Geometry: final body of the model. Coordinates: model frame, mm. Face numbers are marked on the shaded views. A direction names the side the tool comes from. Coordinates: 2 decimals unless noted, no trailing zeros. Order: outer loops, then holes, each group sorted by start corner. A loop starts at its lowest first (then second) coordinate and runs counter-clockwise, first axis right, second up. Notation, with made-up numbers: M -38,-19 L -3,-19 A21 ccw -3,-2 Z; hole C 27.5,86.5 d9. An arc over 180 degrees is marked long. One line per question, with ' | ' between items.
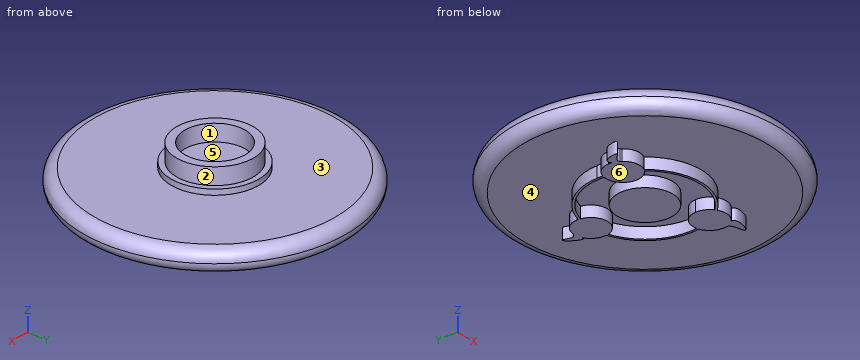
from build123d import *

# Parameters (mm, degrees)
SKETCH1_R           = 12
BOSS_EXTRUDE1_DEPTH = 2
SKETCH2_R           = 3.5
SKETCH2_R_2         = 2.75
BOSS_EXTRUDE2_DEPTH = 2
FILLET1_R           = 1
SKETCH3_R           = 2.5
BOSS_EXTRUDE3_DEPTH = 1
SKETCH4_R           = 3.992210858
BOSS_EXTRUDE4_DEPTH = 0.5


with BuildPart() as part:
    # Sketch1 → Boss-Extrude1 (new body)
    with BuildSketch(Plane.XY):
        Circle(SKETCH1_R)
    extrude(amount=BOSS_EXTRUDE1_DEPTH)

    # Sketch2 → Boss-Extrude2 (add)
    with BuildSketch(Plane.XY.offset(2)):
        Circle(SKETCH2_R)
        Circle(SKETCH2_R_2, mode=Mode.SUBTRACT)
    extrude(amount=BOSS_EXTRUDE2_DEPTH)

    # Fillet1
    fillet1_edges = [part.edges().sort_by_distance(p)[0] for p in [
        (-12, 0, 0),
        (-12, 0, 2),
    ]]
    fillet(fillet1_edges, radius=FILLET1_R - 0.0001)  # a hair under: the kernel refuses the full size

    # Sketch3 → Boss-Extrude3 (add)
    with BuildSketch(Plane(origin=(0, 0, 0), x_dir=(-1, 0, 0), z_dir=(0, 0, -1))):
        with Locations(Location((0, 0, 0), (0, 0, 180))):
            Circle(SKETCH3_R)
        with BuildLine():
            ThreePointArc((-5.067307925, -0.57653308), (-5.873937117, -1.230891086), (-6.062099925, -2.252375207))
            ThreePointArc((-6.062099925, -2.252375207), (-5.915680958, -2.687087026), (-5.644734338, -3.057223228))
            ThreePointArc((-5.644734338, -3.057223228), (-4.802200561, -3.480618607), (-3.873470329, -3.317563506))
            ThreePointArc((-3.873470329, -3.317563506), (-4.675755649, -2.036494318), (-5.067307925, -0.57653308))
        make_face()
        with BuildLine():
            ThreePointArc((-5.644734338, -3.057223228), (-5.915680958, -2.687087026), (-6.062099925, -2.252375207))
            add(Edge.make_bspline(
                [(-6.062099925, -2.252375207), (-6.026517589, -2.751047072), (-8.759907871, -2.687863498), (-5.681591245, -3.687002551), (-5.644734338, -3.057223228)],
                knots=[0, 0, 0, 0, 0.44427951, 1, 1, 1, 1], degree=3))
        make_face()
        with BuildLine():
            ThreePointArc((-1.49486588, 4.876), (-4.265918484, 2.794984703), (-5.067307925, -0.57653308))
            ThreePointArc((-5.067307925, -0.57653308), (-4.970460995, -0.547182079), (-4.871855436, -0.524427893))
            ThreePointArc((-4.871855436, -0.524427893), (-4.098627563, 2.68537746), (-1.464590045, 4.676))
            ThreePointArc((-1.464590045, 4.676), (-1.483103113, 4.775489073), (-1.49486588, 4.876))
        make_face()
        with BuildLine():
            ThreePointArc((-4.871855436, -0.524427893), (-4.970460995, -0.547182079), (-5.067307925, -0.57653308))
            ThreePointArc((-5.067307925, -0.57653308), (-4.675755649, -2.036494318), (-3.873470329, -3.317563506))
            ThreePointArc((-3.873470329, -3.317563506), (-3.786017441, -3.266643945), (-3.702196885, -3.209943649))
            ThreePointArc((-3.702196885, -3.209943649), (-4.492392683, -1.956631796), (-4.871855436, -0.524427893))
        make_face()
        with BuildLine():
            ThreePointArc((-3.702196885, -3.209943649), (-3.786017441, -3.266643945), (-3.873470329, -3.317563506))
            ThreePointArc((-3.873470329, -3.317563506), (0.01581793, -5.09997547), (3.893974917, -3.293472232))
            ThreePointArc((3.893974917, -3.293472232), (3.806118362, -3.243200717), (3.721809355, -3.187182945))
            ThreePointArc((3.721809355, -3.187182945), (0.015022472, -4.899976972), (-3.702196885, -3.209943649))
        make_face()
        with BuildLine():
            ThreePointArc((-3.084074166, -1.996563057), (-3.630573223, -0.838618346), (-4.871855436, -0.524427893))
            ThreePointArc((-4.871855436, -0.524427893), (-4.492392683, -1.956631796), (-3.702196885, -3.209943649))
            ThreePointArc((-3.702196885, -3.209943649), (-3.247508432, -2.677438992), (-3.084074166, -1.996563057))
        make_face()
        with BuildLine():
            ThreePointArc((1.49486588, 4.876), (0, 5.1), (-1.49486588, 4.876))
            ThreePointArc((-1.49486588, 4.876), (-1.483103113, 4.775489073), (-1.464590045, 4.676))
            ThreePointArc((-1.464590045, 4.676), (0, 4.9), (1.464590045, 4.676))
            ThreePointArc((1.464590045, 4.676), (1.483103113, 4.775489073), (1.49486588, 4.876))
        make_face()
        with BuildLine():
            ThreePointArc((-0.554469126, 6.393758942), (-1.275084916, 5.790036997), (-1.49486588, 4.876))
            ThreePointArc((-1.49486588, 4.876), (0, 5.1), (1.49486588, 4.876))
            ThreePointArc((1.49486588, 4.876), (1.49871592, 4.937946879), (1.5, 5))
            ThreePointArc((1.5, 5), (1.10747264, 6.011683919), (0.135327531, 6.493883014))
            ThreePointArc((0.135327531, 6.493883014), (-0.215467229, 6.484443961), (-0.554469126, 6.393758942))
        make_face()
        with BuildLine():
            ThreePointArc((5.074434577, -0.510013455), (4.695210635, -1.991230046), (3.893974917, -3.293472232))
            ThreePointArc((3.893974917, -3.293472232), (4.908886749, -3.438287773), (5.784206585, -2.904590527))
            add(Edge.make_bspline(
                [(5.865406446, -2.794015708), (5.836751545, -2.820305024), (5.809552866, -2.856598637), (5.784206585, -2.904590527)],
                knots=[0.961955758, 0.961955758, 0.961955758, 0.961955758, 1, 1, 1, 1], degree=3))
            ThreePointArc((5.865406446, -2.794015708), (6.004314758, -2.534169766), (6.090380192, -2.252375207))
            ThreePointArc((6.090380192, -2.252375207), (6.112856484, -2.103028092), (6.120373409, -1.952186319))
            ThreePointArc((6.120373409, -1.952186319), (5.831362343, -1.061421113), (5.074434577, -0.510013455))
        make_face()
        with BuildLine():
            ThreePointArc((3.721809355, -3.187182945), (3.806118362, -3.243200717), (3.893974917, -3.293472232))
            ThreePointArc((3.893974917, -3.293472232), (4.695210635, -1.991230046), (5.074434577, -0.510013455))
            ThreePointArc((5.074434577, -0.510013455), (4.97722395, -0.481798325), (4.878348324, -0.460127837))
            ThreePointArc((4.878348324, -0.460127837), (4.511084728, -1.913142593), (3.721809355, -3.187182945))
        make_face()
        with BuildLine():
            ThreePointArc((1.464590045, 4.676), (0, 4.9), (-1.464590045, 4.676))
            ThreePointArc((-1.464590045, 4.676), (0, 3.5), (1.464590045, 4.676))
        make_face()
        with BuildLine():
            add(Edge.make_bspline(
                [(-0.554469126, 6.393758942), (-1.437590662, 6.09502869), (0.002600213, 8.079848895), (-0.001852582, 7.193488902), (-0.442267062, 6.868197163), (0.135327531, 6.493883014)],
                knots=[0, 0, 0, 0, 0.556265111, 0.561970103, 1, 1, 1, 1], degree=3))
            ThreePointArc((-0.554469126, 6.393758942), (-0.215467229, 6.484443961), (0.135327531, 6.493883014))
        make_face()
        with BuildLine():
            ThreePointArc((5.1, 0), (4.100842352, 3.032011215), (1.49486588, 4.876))
            ThreePointArc((1.49486588, 4.876), (1.483103113, 4.775489073), (1.464590045, 4.676))
            ThreePointArc((1.464590045, 4.676), (3.948828385, 2.901164316), (4.9, 0))
            ThreePointArc((4.9, 0), (4.894584088, -0.230318487), (4.878348324, -0.460127837))
            ThreePointArc((4.878348324, -0.460127837), (4.97722395, -0.481798325), (5.074434577, -0.510013455))
            ThreePointArc((5.074434577, -0.510013455), (5.093604634, -0.255326906), (5.1, 0))
        make_face()
        with BuildLine():
            ThreePointArc((4.878348324, -0.460127837), (3.206344863, -1.359804857), (3.721809355, -3.187182945))
            ThreePointArc((3.721809355, -3.187182945), (4.511084728, -1.913142593), (4.878348324, -0.460127837))
        make_face()
        with BuildLine():
            ThreePointArc((6.090380192, -2.252375207), (6.004314758, -2.534169766), (5.865406446, -2.794015708))
            add(Edge.make_bspline(
                [(6.090380192, -2.252375207), (6.684980611, -1.62456302), (7.266645295, -4.471941038), (6.161555953, -2.52231461), (5.865406446, -2.794015708)],
                knots=[0, 0, 0, 0, 0.568767056, 0.961955758, 0.961955758, 0.961955758, 0.961955758], degree=3))
        make_face()
    extrude(amount=BOSS_EXTRUDE3_DEPTH)

    # Sketch4 → Boss-Extrude4 (add)
    with BuildSketch(Plane.XY.offset(2)):
        Circle(SKETCH4_R)
    extrude(amount=BOSS_EXTRUDE4_DEPTH)


solid = part.part
1. Pin query (flat end, axial travel): P1, Ø4, axis at x = -8, y = -6, coming from the -Z side; P2, Ø1.5, axis at x = -0.5, z = -0.5, coming from the -Y side; P3, Ø3, axis at x = 0.5, z = 3, coming from the +Y side. Return the tip coordinate at first contact, or that it passes through.
Response values:
P1: stops at z = 0 | P2: stops at y = -11.65 | P3: stops at y = 11.86
2. Section A-A, the plane z = 3.6. Output: boundary loops of the cut face in (x, y), and give its area (3 significant figures).
Response values:
outline: C 0,0 d7; hole C 0,0 d5.5 | area: 14.7 mm^2
3. Draft query along X for the marked faces 1, 2 and 3. Return one class per face: pulls with the +X half, pulls with the -X half, needs draft (parallel to the pull), parting line crosses it, or undercut.
Response values:
face 1: undercut | face 2: parting line crosses it | face 3: needs draft
4. Section B-B, the plane z = 1.5. Output: boundary loops of the cut face in (x, y), and give its area (3 significant figures).
Response values:
outline: C 0,0 d23.73 | area: 442 mm^2
5. Material intervals for line 1 (X direction, y = 0, z = 2.9); line 2 (X direction, y = 2, z = -0.3), sorted ascending. Write a range as [from, to].
Response values:
line 1: x = [-3.5, -2.75], [2.75, 3.5] | line 2: x = [-4.69, -4.47], [-1.5, 1.5], [4.47, 4.69]
6. Access query for the marked faces 4, 5 and 6. Directions: +Z, -Z, +X, -X, +Y, -Y. A direction counts if a zero-diameter tool reaches every point of the face in a straight line with its end or side. Return the directions, or none.
Response values:
face 4: -Z | face 5: +Z | face 6: -Z, +X, -X, +Y, -Y
